Geometry: final body of the model. Coordinates: model frame, mm. A direction names the side the tool comes from. Coordinates: 2 decimals unless noted, no trailing zeros. Order: outer loops, then holes, each group sorted by start corner. A loop starts at its lowest first (then second) coordinate and runs counter-clockwise, first axis right, second up. Notation, with made-up numbers: M 67,-5.5 L 76,-5.5 A8 ccw 76,1.5 Z; hole C -31.5,0 d2. An arc over 180 degrees is marked long. Use CSV: the item, a comma, the result in double quotes. Start each with the question number.
1. Section query A-A on x = 11. State how many separate pieces and enclosed holes the cut face has, and give its area (3 significant figures).
2. Pull-direction query (Z, two-part tool) for faces 3 (the cylindrical face through (16.3, -80, 0.1)), 4 (the flat face through (28, -1, 49.491)), 5 (the flat face through (0, -1, 1)); classes: pulls with the +Z half, pulls with the -Z half, needs draft (parallel to the pull), parting line crosses it, or undercut.
3. Section query B-B on x = 46.5. Return the cut outline in (y, z), and give its area (3 significant figures).
4. Material intervals for line 1 (Z direction, x = 50, y = 78); line 2 (Y direction, x = 47.5, z = -21); line 3 (Z direction, x = 12, y = -51.5), sorted ascending.
5. Section query C-C on y = 0. Return the cut outline in (x, z) (3 decimals).
6. Section query D-D on z = -42. Return the cut outline in (x, y).
7. Set-up query: faces 1 (the flat face through (28, -1, -49.491)), 2 (the flat face through (33, -1, 44.411)). Return all of +Z, -Z, +X, -X, +Y, -Y with unobstructed straight access to the full face (end or side cutting, diameter ignored); none if empty.
8. First-contact query: P1, Ø3, axis at y = -22.5, z = 0.5, coming from the +X side; P2, Ø12, axis at y = -38.5, z = 36, coming from the -X side. Flat tips, straight axial feed; report the tip coordinate or a pass-through.
from build123d import *

# Parameters (mm, degrees)
F0_W     = 196.053922
F0_H     = 98.98296
F1_DEPTH = 60.96
F2_R     = 5.08
F3_W     = 185.893922
F3_H     = 88.82296
F4_DEPTH = 57.15
F6_R     = 3.175
F6_R_2   = 2.606289
F7_DEPTH = 25.4


with BuildPart() as f1:
    # F0 (on Right) → F1 (new body)
    with BuildSketch(Plane.YZ):
        Rectangle(F0_W, F0_H)
    extrude(amount=F1_DEPTH)

    # F2
    f2_edges = [f1.edges().sort_by_distance(p)[0] for p in [
        (60.96, 98.026961, 0),
        (60.96, 0, 49.49148),
        (60.96, -98.026961, 0),
        (60.96, 0, -49.49148),
    ]]
    fillet(f2_edges, radius=F2_R)

    # F3 (on face) → F4 (cut)
    with BuildSketch(Plane.YZ.offset(60.96)):
        Rectangle(F3_W, F3_H)
    extrude(amount=-F4_DEPTH, mode=Mode.SUBTRACT)

    # F6 (on face) → F7 (join)
    with BuildSketch(Plane.YZ.offset(3.81)):
        Circle(F6_R)
        with Locations((23.48576, 0)):
            Circle(F6_R)
        with Locations((49.327695, 0)):
            Circle(F6_R)
        with Locations((76.993772, 0)):
            Circle(F6_R)
        with Locations((-22.421679, 0)):
            Circle(F6_R)
        with Locations((-50.087753, 0)):
            Circle(F6_R)
        with Locations((-77.395896, 0)):
            Circle(F6_R_2)
    extrude(amount=F7_DEPTH)


solid = f1.part
Results list:
1,separate pieces,"8"
1,enclosed holes,"1"
1,area,"3,110 mm²"
2,face 3,"undercut"
2,face 4,"pulls with the +Z half"
2,face 5,"needs draft"
3,outline,"M -98.03,-49.49 L 98.03,-49.49 L 98.03,49.49 L -98.03,49.49 Z; hole M -92.95,-44.41 L 92.95,-44.41 L 92.95,44.41 L -92.95,44.41 Z"
3,area,"2,890 mm²"
4,line 1,"z = -49.49 to -44.41, 44.41 to 49.49"
4,line 2,"y = -98.03 to -92.95, 92.95 to 98.03"
4,line 3,"z = -49.49 to -44.41, -2.84 to 2.84, 44.41 to 49.49"
5,outline,"M 0,-49.491 L 55.88,-49.491 A5.08 ccw 60.96,-44.411 L 3.81,-44.411 L 3.81,-3.175 L 29.21,-3.175 L 29.21,3.175 L 3.81,3.175 L 3.81,44.411 L 60.96,44.411 A5.08 ccw 55.88,49.491 L 0,49.491 Z"
6,outline,"M 0,-98.03 L 55.88,-98.03 A5.08 ccw 60.96,-92.95 L 3.81,-92.95 L 3.81,92.95 L 60.96,92.95 A5.08 ccw 55.88,98.03 L 0,98.03 Z"
7,face 1,"-Z, +X, -X, +Y, -Y"
7,face 2,"+X"
8,P1,"stops at x = 29.21"
8,P2,"stops at x = 0"
